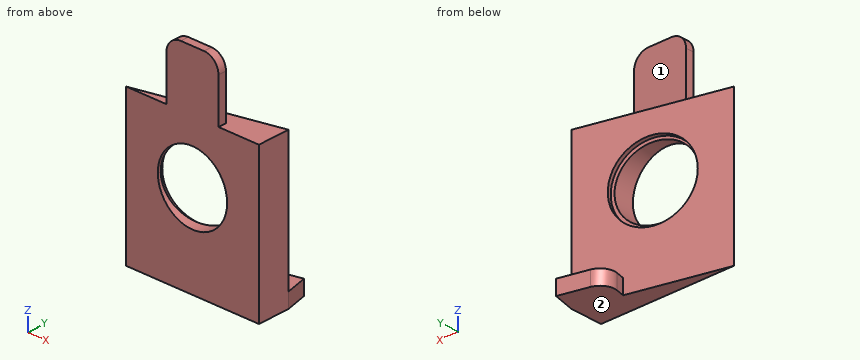
```python
from build123d import *

# Parameters (mm, degrees)
F1_DEPTH = 51.5
F2_R     = 12
F3_DEPTH = 11.001
F4_R     = 13.1
F5_DEPTH = 1.5
F6_W     = 15
F6_H     = 5
F7_DEPTH = 8
F8_W     = 18
F8_H     = 2.8
F9_DEPTH = 20
F10_R    = 5


with BuildPart() as f1:
    # F0 (on Top) → F1 (new body)
    with BuildSketch(Plane.XY):
        Polygon((23, 11), (-23, 0), (23, 0), align=None)
    extrude(amount=F1_DEPTH)

    # F2 (on face) → F3 (cut, through all)
    with BuildSketch(Plane.XZ):
        with Locations((0, 30.75)):
            Circle(F2_R)
    extrude(amount=-F3_DEPTH, mode=Mode.SUBTRACT)

    # F4 (on face) → F5 (cut)
    with BuildSketch(Plane(origin=(-1.2440768887, 5.2025033527, 0), x_dir=(-0.9725788917, -0.2325732132, 0), z_dir=(-0.2325732132, 0.9725788917, 0))):
        with Locations((-1.2791526727, 30.75)):
            Circle(F4_R)
    extrude(amount=-F5_DEPTH, mode=Mode.SUBTRACT)

    # F6 (on face) → F7 (join)
    with BuildSketch(Plane(origin=(-1.2440768887, 5.2025033527, 0), x_dir=(-0.9725788917, -0.2325732132, 0), z_dir=(-0.2325732132, 0.9725788917, 0))):
        with Locations((-17.4276198535, 2.5)):
            Rectangle(F6_W, F6_H)
    extrude(amount=F7_DEPTH)

    # F8 (on face) → F9 (join)
    with BuildSketch(Plane.XY.offset(51.5)):
        with Locations((0, 1.4)):
            Rectangle(F8_W, F8_H)
    extrude(amount=F9_DEPTH)

    # F10
    f10_edges = [f1.edges().sort_by_distance(p)[0] for p in [
        (6.550731, 15.292033, 2.5),
        (-9, 1.4, 71.5),
        (9, 1.4, 71.5),
    ]]
    fillet(f10_edges, radius=F10_R)


solid = f1.part
```
Read the model definition and answer for the solid it produces. Units are mm, in the model's axes. Face numbers are marked on the shaded views. A direction names the side the tool comes from. Give positions to 0.01 mm unless a question says otherwise; leave off trailing zeros. Write each loop counter-clockwise with the first axis right and the second up, starting at its lowest first coordinate (ties: lowest second). Pieces come first, ordered by that corner, then holes. Notation, with made-up numbers: M 26,-37 L 46,-37 A32 cw 46,-8 Z; hole C -19,83 d4. An arc over 180 degrees is marked long. Put each result on its own line as item: value. Start each with the question number.
1. The part is cut by section D-D, the plane y = 12.5. Give the vertices of the cut face in (x, z), and give its area (3 significant figures).
2. Consider line 1 along Z through (x, y) = (0, 5.25); line 2 along X through (y, z) = (3.75, 30.75); line 3 along Z through (x, y) = (0, 1.75). Determine where each line is inside the solid, lowest interval first.
3. The part is cut by section C-C, the plane x = 17. Give the vertices of the cut face in (y, z).
4. The part is cut by section B-B, the plane z = 63. Give the vertices of the cut face in (x, y).
5. Which of the six approach directions +Z, -Z, +X, -X, +Y, -Y give full straight-line access (tool end or side, diameter ignored) to the marked faces 1 and 2?
6. The part is cut by section A-A, the plane z = 34. Give the vertices of the cut face in (x, y), and give its area (3 significant figures).
7. Each of these flat-tipped pins is pushed along its axis until it touches: pin 1 Ø9 at (x, y) = (11, 4) entering from +Z; pin 2 Ø1.5 at (x, z) = (-9, 56.5) entering from -Y; pin 3 Ø10 at (y, z) = (4.5, 57) entering from -X; pin 4 Ø3.5 at (x, y) = (12.5, 14.5) entering from +Z. Where does it stop, or does it pass through?
Final values:
1. outline: M 7.66,0 L 22.64,0 L 22.64,5 L 7.66,5 Z
1. area: 74.9 mm²
2. line 1: z = 0 to 17.65, 43.85 to 51.5
2. line 2: x = 12 to 23
2. line 3: z = 0 to 18.75, 42.75 to 71.5
3. outline: M 0,0 L 17.79,0 L 17.79,5 L 9.57,5 L 9.57,51.5 L 0,51.5 Z
4. outline: M -9,0 L 9,0 L 9,2.8 L -9,2.8 Z
5. face 1: +Z, +X, -X, +Y
5. face 2: -Z, +X, -X, +Y, -Y
6. outline: M -23,0 L -11.55,0 L -11.55,1.2 L -11.99,1.09 L -12.34,2.55 Z; M 11.55,0 L 23,0 L 23,11 L 12.34,8.45 L 12.69,6.99 L 11.55,6.72 Z
6. area: 123 mm²
7. pin 1: stops at z = 70.73
7. pin 2: stops at y = 0
7. pin 3: stops at x = -9
7. pin 4: stops at z = 5
